Design review of the part shown in the three views and the two pictorial views. Dimensions are in mm from the part's minimum x, y and z. A direction names the side the tool comes from. Round coordinates to 2 decimals unless told otherwise and drop trailing zeros. Loops run counter-clockwise (first coordinate to the right, second up) from the corner with the lowest first, then second, coordinate; pieces in that order, holes last. Notation, with made-up numbers: (30, 17.25) -> (43, 17.25) arc R16 ccw to (43, 24.25) -> close; hole circle Ø10 at (-26.75, 86). An arc over 180 degrees is marked (long way). Write each question's results on one line, items separated by ' | '. Start each with the question number.
Item 1: For L1, parallel to Y at x = 47.9, z = 22.5; L2, parallel to Y at x = 26.5, z = 11; L3, parallel to X at y = 9, z = 33, list the stretches that pass through material, from the lowest coordinate up. Write a range as from..to.
Item 2: Clearance check with flat-ended pins moving along their axes: pin 1 Ø3 at (x, z) = (20, 13) entering from +Y; pin 2 Ø1.5 at (y, z) = (40.5, 19.5) entering from -X. State where each tip first meets the part, or that it passes through.
Item 3: We need section B-B (z = 22.5). Give the boundary of the cut face in (x, y), and give its area (3 significant figures).
Item 4: Tool access review of the marked faces 4 and 5: name each direction out of +Z, -Z, +X, -X, +Y, -Y from which nothing blocks a thin tool from reaching the whole face with its end or side.
Item 5: We need section C-C (x = 22.5). Give the boundary of the cut face in (y, z).
Item 6: Mouldability with a two-part tool opening along Z and no side actions: class the marked faces 1, 2 and 3 as pulls with the +Z half, pulls with the -Z half, needs draft (parallel to the pull), parting line crosses it, or undercut.
Item 7: We need section D-D (y = 8.5). Give the boundary of the cut face in (x, z), and give its area (3 significant figures).
Item 8: We need section A-A (y = 22). Give the boundary of the cut face in (x, z).
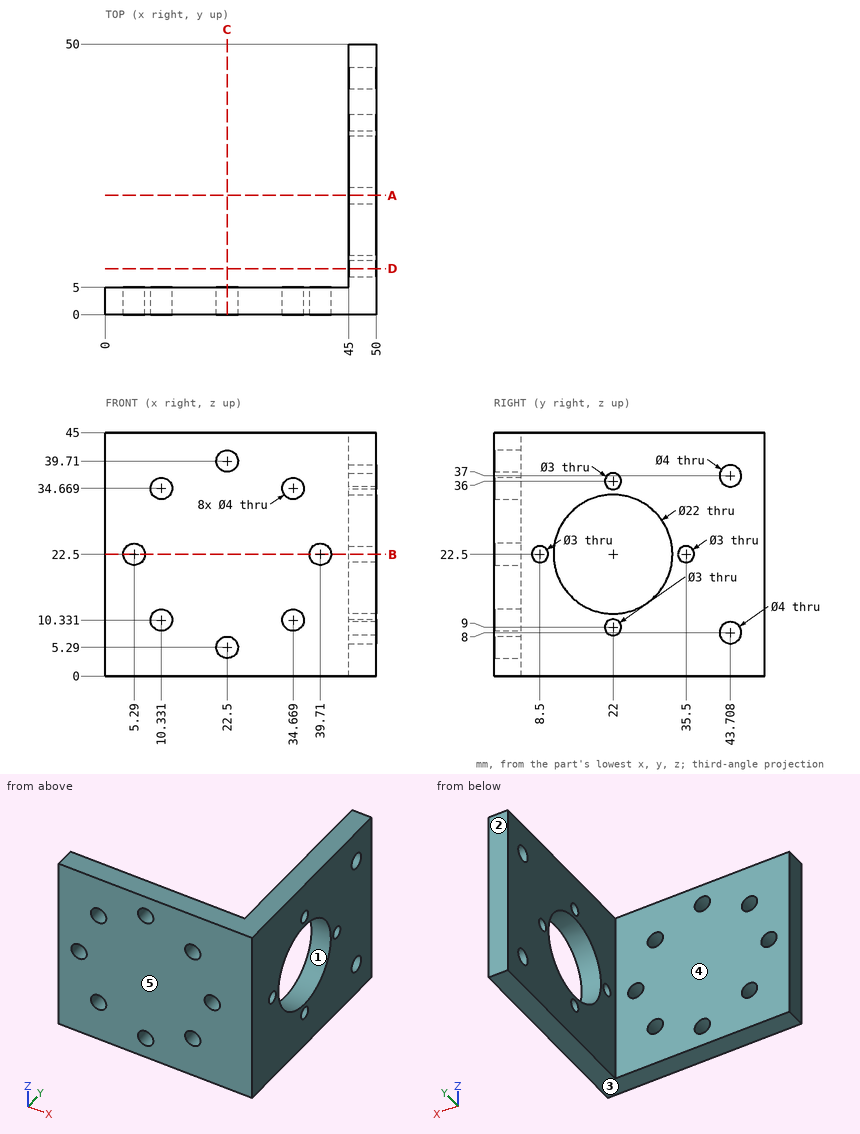
Here are the results:
1) L1: y = 0..7, 10..11, 33..34, 37..50 | L2: y = 0..5 | L3: x = 45..50
2) pin 1: stops at y = 5 | pin 2: stops at x = 45
3) outline: (0, 0) -> (3.29, 0) -> (3.29, 5) -> (0, 5) -> close; (7.29, 0) -> (37.71, 0) -> (37.71, 5) -> (7.29, 5) -> close; (41.71, 0) -> (50, 0) -> (50, 7) -> (45, 7) -> (45, 5) -> (41.71, 5) -> close; (45, 10) -> (50, 10) -> (50, 11) -> (45, 11) -> close; (45, 33) -> (50, 33) -> (50, 34) -> (45, 34) -> close; (45, 37) -> (50, 37) -> (50, 50) -> (45, 50) -> close | area: 295 mm2
4) face 4: +Z, -Z, -X, +Y | face 5: +Z, -Z, +X, -X, -Y
5) outline: (0, 0) -> (5, 0) -> (5, 3.29) -> (0, 3.29) -> close; (0, 7.29) -> (5, 7.29) -> (5, 37.71) -> (0, 37.71) -> close; (0, 41.71) -> (5, 41.71) -> (5, 45) -> (0, 45) -> close
6) face 1: undercut | face 2: needs draft | face 3: pulls with the -Z half
7) outline: (45, 0) -> (50, 0) -> (50, 21) -> (45, 21) -> close; (45, 24) -> (50, 24) -> (50, 45) -> (45, 45) -> close | area: 210 mm2
8) outline: (45, 0) -> (50, 0) -> (50, 7.5) -> (45, 7.5) -> close; (45, 10.5) -> (50, 10.5) -> (50, 11.5) -> (45, 11.5) -> close; (45, 33.5) -> (50, 33.5) -> (50, 34.5) -> (45, 34.5) -> close; (45, 37.5) -> (50, 37.5) -> (50, 45) -> (45, 45) -> close
